Could you check a few things on this model? Use its own coordinates, in mm. Coordinates: 2 decimals unless noted, no trailing zeros. Loops run counter-clockwise (first coordinate to the right, second up) from the corner with the lowest first, then second, coordinate; pieces in that order, holes last. Notation, with made-up numbers: (69, -12) -> (120, -12) arc R15 cw to (120, 7) -> close; hole circle Ø7 at (47.5, -19). An arc over 180 degrees is marked (long way). One line per question, with ' | ' between items. Start each with the question number.
(1) I'm going to push a flat-ended pin straight in: pin 1 Ø20.5 at (x, z) = (-14, 1.5) entering from +Y. Where does the tip first touch, or does it pass through?
(2) Suppose I cut it at D-D (z = 25). Please give me the cut outline in (x, y).
(3) Suppose I cut it at C-C (x = -28). Please give me the cut outline in (y, z), plus the area to 3 significant figures.
(4) If I drill on line 1 along Z through (x, y) = (0, 0.4); line 2 along Y through (x, z) = (1, -24.5); line 3 along X through (y, z) = (1, -8.5), over which ranges is the centre line in solid material (lowest first)?
(5) Suppose I cut it at B-B (y = 4.5). Please give me the cut outline in (x, z).
(6) Suppose I cut it at A-A (x = 0). Please give me the cut outline in (y, z), plus the area to 4 significant figures.
Autodesk Inventor part; units mm, degrees
ref_plane "YZ Plane" through (0, 0, 0) normal (1, 0, 0) x (0, 1, 0)
ref_plane "XZ Plane" through (0, 0, 0) normal (0, 1, 0) x (-1, 0, 0)
ref_plane "XY Plane" through (0, 0, 0) normal (0, 0, 1) x (1, 0, 0)
sketch "Эскиз1" plane through (0, 0, 0) normal (0, 1, 0) x (-1, 0, 0)
  circle A0 centre (0, 0) radius 34
  dimension "d0" = 68
extrude "Выдавливание1" add sketch "Эскиз1" along normal blind 2
sketch "Эскиз2" plane through (0, 2, 0) normal (0, 1, 0) x (1, 0, 0)
  circle A0 centre (0, 0) radius 28
  line L0 (19.5959, -20) -> (19.5959, 20)
  line L1 (19.5959, -20) -> (-28, 0)
  line L2 (19.5959, 20) -> (-28, 0)
  circle A1 centre (-28, 0) radius 2.5
  circle A2 centre (19.5959, -20) radius 2.5
  circle A3 centre (19.5959, 20) radius 2.5
  dimension "d3" = 56
  dimension "d4" = 40
  dimension "d5" = 5
extrude "Выдавливание2" add sketch "Эскиз2" along normal blind 5 contours A3 L0 A0 | A0 A3 | A2 A0 | A0 L0 A2 | L2 A3 A0 | L0 A3 L2 | L1 A2 L0 | A0 A2 L1 | A1 L2 A0 | A0 A1 | A1 L1 L2 | A0 L1 A1
chamfer "Фаска1" distance 0.5 angle 45 3 edges at (17.0959, 7, -20) (17.0959, 7, 20) (-30.5, 7, 0)
sketch "Эскиз3" plane through (0, 2, 0) normal (0, 1, 0) x (1, 0, 0)
  circle A0 centre (0, 0) radius 20
  circle A1 centre (-28, 0) radius 2
  circle A2 centre (19.5959, 20) radius 2
  circle A3 centre (19.5959, -20) radius 2
  line L0 (-28, 0) -> (19.5959, -20)
  circle A4 centre (-28, 0) radius 2.5
  line L1 (19.5959, 20) -> (-28, 0)
  circle A5 centre (11.289, -16.5094) radius 1.5
  circle A6 centre (11.289, 16.5094) radius 1.5
  circle A7 centre (-20, 0) radius 1.5
  dimension "d11" = 40
  dimension "d17" = 3
extrude "Выдавливание3" cut sketch "Эскиз3" against normal blind 5 contours A0 A5 L0 A7 L1 A6 | A6 L1 A0 | A0 L0 A5 | L1 A6 A0 | L1 A0 A6 | A0 A5 L0 | A5 A0 L0 | A7 A0 picked at (11.3081, 15.9275) picked at (11.3081, -15.9275) picked at (10.6892, 16.4081) picked at (-9.3619, 9.1636) picked at (10.6892, -16.4081) picked at (-9.3619, -9.1636) picked at (-19.4958, 0)
chamfer "Фаска2" distance 1.5 angle 45 1 edges at (-20, 2, 0)
sketch "Эскиз4" plane through (0, 2, 0) normal (0, 1, 0) x (1, 0, 0)
  circle A0 centre (-28, 0) radius 2
  circle A1 centre (19.5959, -20) radius 2
  circle A2 centre (19.5959, 20) radius 2
  circle A3 centre (-28, 0) radius 2
  line L0 (19.5959, -20) -> (-28, 0)
  circle A4 centre (19.5959, 20) radius 2
  line L1 (-28, 0) -> (19.5959, 20)
  circle A5 centre (0, 0) radius 20
  circle A6 centre (0, 0) radius 21.5
  circle A7 centre (12.9117, 17.1912) radius 1.5
  circle A8 centre (12.9117, -17.1912) radius 1.5
  circle A9 centre (-21.5, 0) radius 1.5
extrude "Выдавливание4" add sketch "Эскиз4" against normal up to surface (2 mm away) contours A7 L1 A6 | A6 L1 A7 | A9 A6 | A6 A9 | A8 L0 A6 | A6 L0 A8 | A6 A7 L1 | L1 A7 A6 | A6 A8 L0 | L0 A8 A6
properties part number "Шапка лидара"
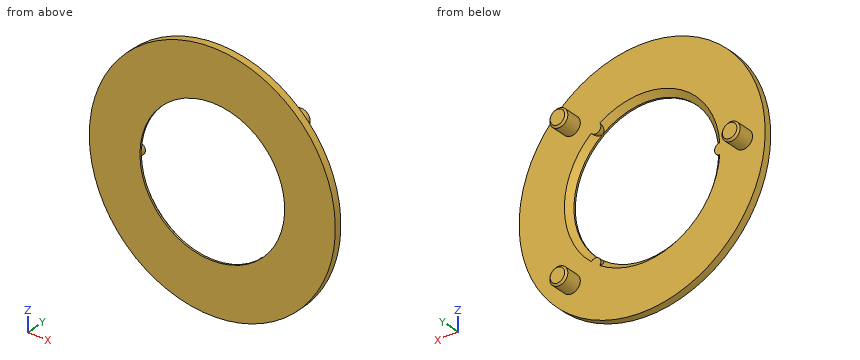
Checks:
1) pin 1: stops at y = 2
2) outline: (-23.04, 0) -> (23.04, 0) -> (23.04, 2) -> (-23.04, 2) -> close
3) outline: (0, -19.29) -> (2, -19.29) -> (2, -2.5) -> (6.5, -2.5) -> (7, -2) -> (7, 2) -> (6.5, 2.5) -> (2, 2.5) -> (2, 19.29) -> (0, 19.29) -> close | area: 102 mm^2
4) line 1: z = -34 to -20, 20 to 34 | line 2: y = 0 to 2 | line 3: x = -32.92 to -18.65, 18.65 to 32.92
5) outline: circle Ø5 at (-28, 0); circle Ø5 at (19.6, -20); circle Ø5 at (19.6, 20)
6) outline: (0, -34) -> (2, -34) -> (2, -21.5) -> (0.5, -20) -> (0, -20) -> close; (0, 20) -> (0.5, 20) -> (2, 21.5) -> (2, 34) -> (0, 34) -> close | area: 53.75 mm^2
